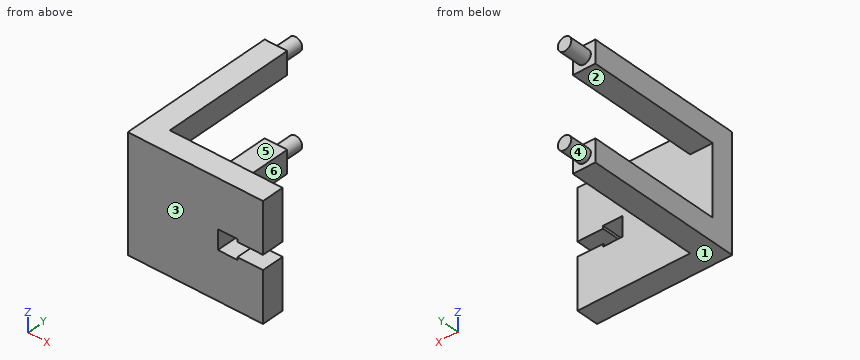
Autodesk Inventor part; units mm, degrees
ref_plane "YZ Plane" through (0, 0, 0) normal (1, 0, 0) x (0, 1, 0)
ref_plane "XZ Plane" through (0, 0, 0) normal (0, 1, 0) x (-1, 0, 0)
ref_plane "XY Plane" through (0, 0, 0) normal (0, 0, 1) x (1, 0, 0)
sketch "Sketch1" plane through (0, 0, 0) normal (0, 1, 0) x (-1, 0, 0)
  line L0 (0, 0) -> (-76.2, 0)
  line L1 (-76.2, 0) -> (-76.2, -64.6684)
  line L2 (-76.2, -64.6684) -> (0, -64.6684)
  line L3 (0, -64.6684) -> (0, 0)
  line L4 (0, -32.3342) -> (-50.8, -32.3342)
  line L5 (-50.8, -32.3342) -> (-50.8, -37.8342)
  line L6 (-50.8, -37.8342) -> (-61.8, -37.8342)
  line L7 (-61.8, -37.8342) -> (-61.8, -26.8342)
  line L8 (-61.8, -26.8342) -> (-50.8, -26.8342)
  line L9 (-50.8, -26.8342) -> (-50.8, -37.8342)
  dimension "d0" = 76.2
  dimension "d1" = 64.6684
  dimension "d2" = 50.8
  dimension "d3" = 5.5
  dimension "d4" = 11
  dimension "d5" = 11
extrude "Extrusion1" add sketch "Sketch1" along normal blind 12.7
sketch "Sketch2" plane through (0, 12.7, 0) normal (0, 1, 0) x (1, 0, 0)
  line L0 (0, 0) -> (76.2, 0)
  line L1 (0, 0) -> (12.7, 0)
  line L2 (12.7, 0) -> (12.7, 12.7)
  line L3 (12.7, 12.7) -> (0, 12.7)
  line L4 (0, 12.7) -> (0, 0)
  line L5 (0, 64.6684) -> (12.7, 64.6684)
  line L6 (12.7, 64.6684) -> (12.7, 51.9684)
  line L7 (12.7, 51.9684) -> (0, 51.9684)
  line L8 (0, 51.9684) -> (0, 64.6684)
  dimension "d8" = 12.7
  dimension "d9" = 12.7
  dimension "d10" = 12.7
  dimension "d11" = 12.7
extrude "Extrusion2" add sketch "Sketch2" along normal blind 76.2
sketch "Sketch3" plane through (0, 88.9, 0) normal (0, 1, 0) x (1, 0, 0)
  line L0 (0, 0) -> (0, 6.35)
  line L1 (0, 64.6684) -> (0, 0)
  line L2 (0, 6.35) -> (6.35, 6.35)
  circle A0 centre (6.35, 6.35) radius 3.81
  line L3 (0, 64.6684) -> (0, 58.3184)
  line L4 (0, 58.3184) -> (6.35, 58.3184)
  circle A1 centre (6.35, 58.3184) radius 3.81
  dimension "d14" = 6.35
  dimension "d15" = 6.35
  dimension "d16" = 7.62
  dimension "d17" = 6.35
  dimension "d18" = 7.62
extrude "Extrusion3" add sketch "Sketch3" along normal blind 12.7
sketch "Sketch4" plane through (0, 0, 0) normal (0, -1, 0) x (1, 0, 0)
  line L0 (76.2, 0) -> (76.2, -64.6684)
  line L1 (76.2, -32.3342) -> (76.2, -36.3342)
  line L2 (76.2, -36.3342) -> (61.8, -36.3342)
  line L3 (61.8, -37.8342) -> (61.8, -26.8342)
  line L4 (76.2, -36.3342) -> (50.8, -36.3342)
  line L5 (50.8, -36.3342) -> (50.8, -28.3332)
  line L6 (50.8, -28.3332) -> (76.2, -28.3332)
  line L7 (76.2, -28.3332) -> (76.2, -36.3342)
  point P0 (0, 0)
  dimension "d21" = 4
  dimension "d22" = 25.4
  dimension "d23" = 8.001
extrude "Extrusion4" cut sketch "Sketch4" against normal blind 12.7
properties part number "Maglev_top"
Could you check a few things on this model? Use its own coordinates, in mm. Face numbers are marked on the shaded views. A direction names the side the tool comes from. Round coordinates to 2 decimals unless told otherwise and drop trailing zeros. Loops run counter-clockwise (first coordinate to the right, second up) from the corner with the lowest first, then second, coordinate; pieces in that order, holes last.
Q1. Thinking about a two-plate mould opening in Z: for the marked faces 1, 2 and 3, which applies, pulls with the +Z half, pulls with the -Z half, needs draft (parallel to the pull), parting line crosses it, or undercut?
Q2. I want a section at B-B (x = 6.35). Write out the boundary of the cut face in (y, z).
Q3. I want a section at D-D (z = -40.5). Write out the boundary of the cut face in (x, y).
Q4. Please list where these lines run through material, in increasing order: L1, parallel to Z at x = 3, y = 44; L2, parallel to Y at x = 35, z = -54.
Q5. For P1, Ø10, axis at y = 50, z = -59.5, coming from the +X side; P2, Ø5.5, axis at y = 3.5, z = -32, coming from the +X side, each with a flat end and sliding along its axis, tell me the tip position at first contact or that it passes through.
Q6. I want a section at C-C (z = -6.35). Write out the boundary of the cut face in (x, y).
Q7. I want a section at A-A (y = 14). Write out the boundary of the cut face in (x, z).
Q8. On a 3-axis mill with a long thin cutter (end or side, diameter ignored), from which of +Z, -Z, +X, -X, +Y, -Y can I reach the whole of each face in a straight line? I mean the marked faces 4, 5 and 6. Say none if no direction works.
Answer below:
1. face 1: pulls with the -Z half
1. face 2: undercut
1. face 3: needs draft
2. outline: (0, -64.67) - (88.9, -64.67) - (88.9, -62.13) - (101.6, -62.13) - (101.6, -54.51) - (88.9, -54.51) - (88.9, -51.97) - (12.7, -51.97) - (12.7, -12.7) - (88.9, -12.7) - (88.9, -10.16) - (101.6, -10.16) - (101.6, -2.54) - (88.9, -2.54) - (88.9, 0) - (0, 0) - close
3. outline: (0, 0) - (76.2, 0) - (76.2, 12.7) - (0, 12.7) - close
4. L1: z = -64.67 to -51.97, -12.7 to 0
4. L2: y = 0 to 12.7
5. P1: stops at x = 12.7
5. P2: stops at x = 50.8
6. outline: (0, 0) - (76.2, 0) - (76.2, 12.7) - (12.7, 12.7) - (12.7, 88.9) - (10.16, 88.9) - (10.16, 101.6) - (2.54, 101.6) - (2.54, 88.9) - (0, 88.9) - close
7. outline: (0, -64.67) - (12.7, -64.67) - (12.7, -51.97) - (0, -51.97) - close; (0, -12.7) - (12.7, -12.7) - (12.7, 0) - (0, 0) - close
8. face 4: +Y
8. face 5: +X, -X, +Y
8. face 6: +Z, -Z, +X, +Y
